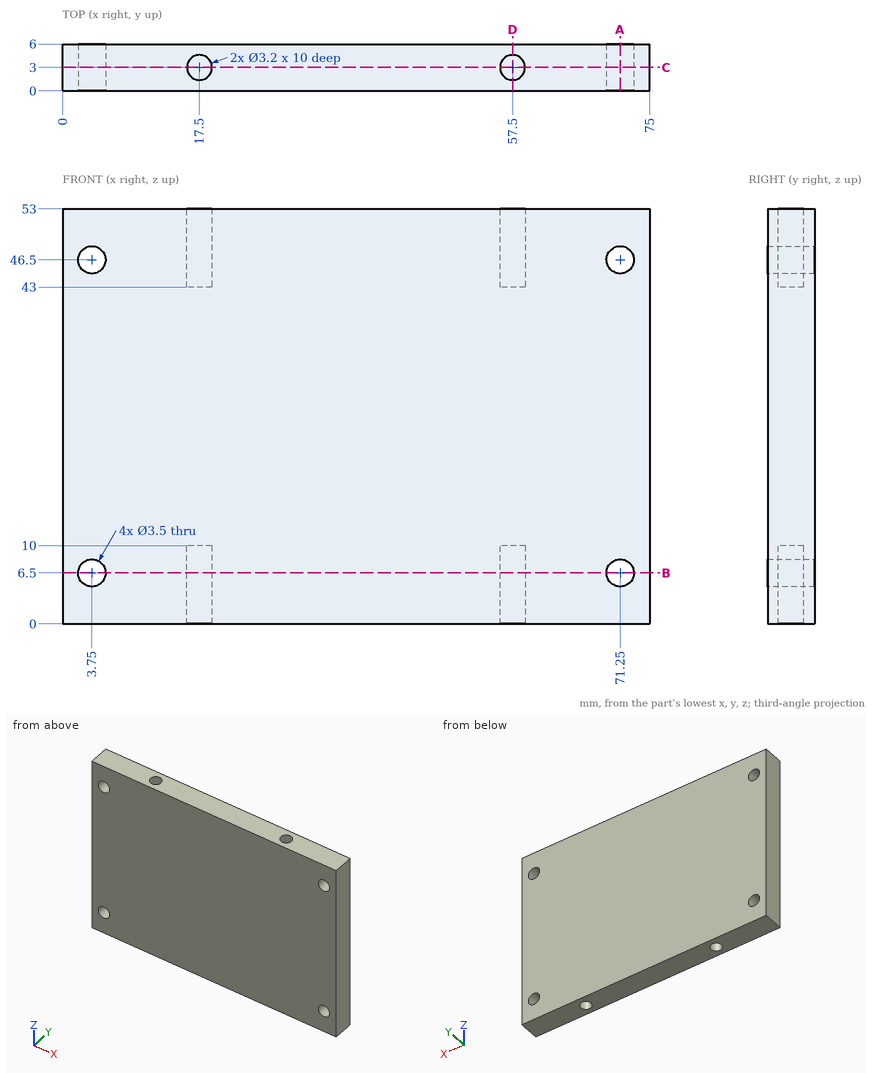
Geometry check sheet. Reference: drawing and pictorial views, mm from the part's lowest x, y, z. Give positions to 0.01 mm unless a question says otherwise; leave off trailing zeros. Order: outer loops, then holes, each group sorted by start corner. A loop starts at its lowest first (then second) coordinate and runs counter-clockwise, first axis right, second up. Notation, with made-up numbers: M 69,-6.5 L 102,-6.5 A14 cw 102,4.5 Z; hole C 35.5,15.25 d7. An arc over 180 degrees is marked long. Answer in a Markdown table with one row per item. Add a question column.
Q1. Sectioned sample at D-D, the plane x = 57.5. Record the boundary of the cut face in (y, z), and give its area (3 significant figures).
Q2. Sectioned sample at B-B, the plane z = 6.5. Record the boundary of the cut face in (x, y).
Q3. Sectioned sample at C-C, the plane y = 3. Record the boundary of the cut face in (x, z).
Q4. Thickness scan on L1, parallel to X at y = 4.2, z = 6.5; L2, parallel to Y at x = 17.5, z = 47.5; L3, parallel to X at y = 2.5, z = 6. Record the ranges inside material, lowest first.
Q5. Gauge pin test, flat ends, axial feed: pin 1 Ø1.6 at (x, y) = (18, 3) entering from -Z; pin 2 Ø3 at (x, z) = (3.75, 46.5) entering from +Y. Record the tip position at first contact, or that the pin passes through.
Q6. Sectioned sample at A-A, the plane x = 71.25. Record the boundary of the cut face in (y, z).
Verdict:
| question | item | result |
|---|---|---|
| 1 | outline | M 0,0 L 1.4,0 L 1.4,10 L 4.6,10 L 4.6,0 L 6,0 L 6,53 L 4.6,53 L 4.6,43 L 1.4,43 L 1.4,53 L 0,53 Z |
| 1 | area | 254 mm² |
| 2 | outline | M 0,0 L 2,0 L 2,6 L 0,6 Z; M 5.5,0 L 69.5,0 L 69.5,6 L 5.5,6 Z; M 73,0 L 75,0 L 75,6 L 73,6 Z; hole C 17.5,3 d3.2; hole C 57.5,3 d3.2 |
| 3 | outline | M 0,0 L 15.9,0 L 15.9,10 L 19.1,10 L 19.1,0 L 55.9,0 L 55.9,10 L 59.1,10 L 59.1,0 L 75,0 L 75,53 L 59.1,53 L 59.1,43 L 55.9,43 L 55.9,53 L 19.1,53 L 19.1,43 L 15.9,43 L 15.9,53 L 0,53 Z; hole C 3.75,6.5 d3.5; hole C 3.75,46.5 d3.5; hole C 71.25,6.5 d3.5; hole C 71.25,46.5 d3.5 |
| 4 | L1 | 0 to 2, 5.5 to 16.44, 18.56 to 56.44, 58.56 to 69.5, 73 to 75 |
| 4 | L2 | 0 to 1.4, 4.6 to 6 |
| 4 | L3 | 0 to 2.07, 5.43 to 15.98, 19.02 to 55.98, 59.02 to 69.57, 72.93 to 75 |
| 5 | pin 1 | z = 10 |
| 5 | pin 2 | through |
| 6 | outline | M 0,0 L 6,0 L 6,4.75 L 0,4.75 Z; M 0,8.25 L 6,8.25 L 6,44.75 L 0,44.75 Z; M 0,48.25 L 6,48.25 L 6,53 L 0,53 Z |
